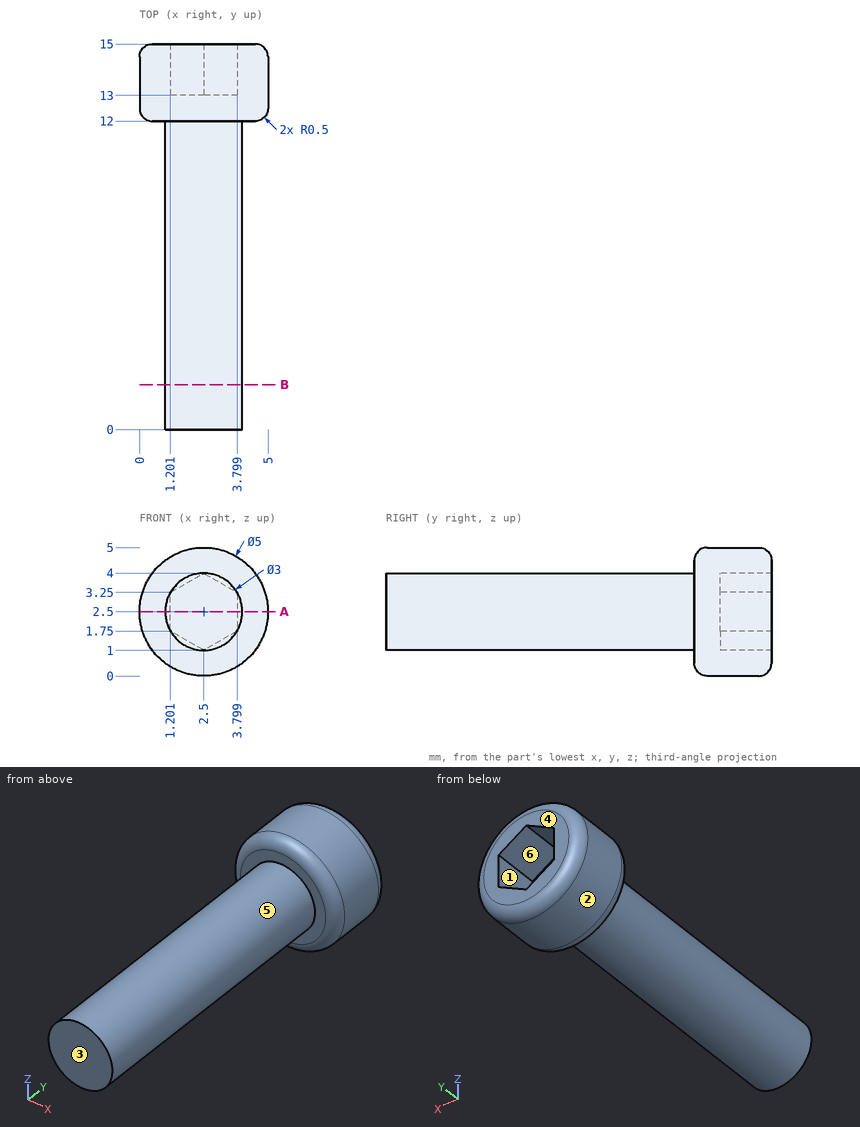
Part print with two shaded views. Sizes in mm from the minimum x, y, z corner. A direction names the side the tool comes from. Round coordinates to 2 decimals unless told otherwise and drop trailing zeros. Write each loop counter-clockwise with the first axis right and the second up, starting at its lowest first coordinate (ties: lowest second). Pieces come first, ordered by that corner, then holes. Notation, with made-up numbers: (33.5, 83) -> (41.5, 83) arc R21 cw to (41.5, 117) -> close; hole circle Ø10 at (-35, -29). An arc over 180 degrees is marked (long way). Use one line per item in the form item = value.
Q1. Tool access for the marked faces 4, 5 and 6: list every direction of +Z, -Z, +X, -X, +Y, -Y with a clear straight run to the whole face (end or side of a thin tool).
Conclusion:
face_4 = +Z, -Z, +X, -X, +Y
face_5 = -Y
face_6 = +Y
Q2. Drill centre lines: L1, parallel to Y at x = 3.55, z = 4.1; L2, parallel to X at y = 1, z = 2.5; L3, parallel to Z at x = 3.8, y = 5. Where is each one in solid material? Low to high.
Conclusion:
L1 = 12 to 15
L2 = 1 to 4
L3 = 1.75 to 3.25
Q3. Band-saw the part on B-B, the plane y = 1.75. Write the cut outline in (x, z), then the cut area to 3 significant figures.
Conclusion:
outline = circle Ø3 at (2.5, 2.5)
area = 7.07 mm²
Q4. Band-saw the part on A-A, the plane z = 2.5. Write the cut outline in (x, y).
Conclusion:
outline = (0, 12.5) arc R0.5 ccw to (0.5, 12) -> (1, 12) -> (1, 0) -> (4, 0) -> (4, 12) -> (4.5, 12) arc R0.5 ccw to (5, 12.5) -> (5, 14.5) arc R0.5 ccw to (4.5, 15) -> (3.8, 15) -> (3.8, 13) -> (1.2, 13) -> (1.2, 15) -> (0.5, 15) arc R0.5 ccw to (0, 14.5) -> close
Q5. Drop flat-ended pins along their axis: P1, Ø0.8, axis at x = 3, z = 2.5, coming from the +Y side; P2, Ø3, axis at y = 4.5, z = 2.5, coming from the -X side; P3, Ø1, axis at x = 3, y = 8, coming from the +Z side. Give the stop position or say it passes through.
Conclusion:
P1 = 13
P2 = 1
P3 = 4
Q6. Two-plate mould, pull along X, no slides. Class the marked faces 1, 2 and 3: released by +X, released by -X, zero draft, split by the parting line, or undercut.
Conclusion:
face_1 = undercut
face_2 = split by the parting line
face_3 = zero draft
